Could you check a few things on this model? Use its own coordinates, in mm. Round coordinates to 2 decimals unless told otherwise and drop trailing zeros. Loops run counter-clockwise (first coordinate to the right, second up) from the corner with the lowest first, then second, coordinate; pieces in that order, holes last. Notation, with made-up numbers: M 86.25,58 L 90.25,58 A10 cw 90.25,68 Z; hole C -17.75,-27 d4. An arc over 180 degrees is marked long. Answer in a Markdown table with one row per item.
```python
from build123d import *

# Parameters (mm, degrees)
SKETCH1_R           = 40
SKETCH1_R_2         = 4.1
SKETCH1_R_3         = 1
SKETCH1_R_4         = 2.5
BOSS_EXTRUDE1_DEPTH = 3.175


with BuildPart() as part:
    # Sketch1 → Boss-Extrude1 (new body)
    with BuildSketch(Plane.XY):
        Circle(SKETCH1_R)
        Circle(SKETCH1_R_2, mode=Mode.SUBTRACT)
        with Locations((10, 0)):
            Circle(SKETCH1_R_3, mode=Mode.SUBTRACT)
        with Locations((0, -10)):
            Circle(SKETCH1_R_3, mode=Mode.SUBTRACT)
        with Locations((-10, 0)):
            Circle(SKETCH1_R_3, mode=Mode.SUBTRACT)
        with Locations((0, 10)):
            Circle(SKETCH1_R_3, mode=Mode.SUBTRACT)
        with Locations((0, 32.500000024)):
            Circle(SKETCH1_R_4, mode=Mode.SUBTRACT)
        with Locations((32.500000024, 0)):
            Circle(SKETCH1_R_4, mode=Mode.SUBTRACT)
        with Locations((0, -32.500000024)):
            Circle(SKETCH1_R_4, mode=Mode.SUBTRACT)
        with Locations((-32.500000024, 0)):
            Circle(SKETCH1_R_4, mode=Mode.SUBTRACT)
        with BuildLine():
            ThreePointArc((1.892882879, 15.429065651), (16.987986018, 13.094493375), (30.244053834, 5.505749571))
            ThreePointArc((30.244053834, 5.505749571), (30.545302534, 3.644891179), (28.754168977, 3.057196265))
            ThreePointArc((28.754168977, 3.057196265), (16.369486394, 10.54396404), (2.033129259, 12.519038334))
            ThreePointArc((2.033129259, 12.519038334), (0.481040246, 13.902629865), (1.892882879, 15.429065651))
        make_face(mode=Mode.SUBTRACT)
        with BuildLine():
            ThreePointArc((15.429065651, -1.892882879), (13.094493375, -16.987986018), (5.505749571, -30.244053834))
            ThreePointArc((5.505749571, -30.244053834), (3.644891179, -30.545302534), (3.057196265, -28.754168977))
            ThreePointArc((3.057196265, -28.754168977), (10.54396404, -16.369486394), (12.519038334, -2.033129259))
            ThreePointArc((12.519038334, -2.033129259), (13.902629865, -0.481040246), (15.429065651, -1.892882879))
        make_face(mode=Mode.SUBTRACT)
        with BuildLine():
            ThreePointArc((-1.892882879, -15.429065651), (-16.987986018, -13.094493375), (-30.244053834, -5.505749571))
            ThreePointArc((-30.244053834, -5.505749571), (-30.545302534, -3.644891179), (-28.754168977, -3.057196265))
            ThreePointArc((-28.754168977, -3.057196265), (-16.369486394, -10.54396404), (-2.033129259, -12.519038334))
            ThreePointArc((-2.033129259, -12.519038334), (-0.481040246, -13.902629865), (-1.892882879, -15.429065651))
        make_face(mode=Mode.SUBTRACT)
        with BuildLine():
            ThreePointArc((-15.429065651, 1.892882879), (-13.094493375, 16.987986018), (-5.505749571, 30.244053834))
            ThreePointArc((-5.505749571, 30.244053834), (-3.644891179, 30.545302534), (-3.057196265, 28.754168977))
            ThreePointArc((-3.057196265, 28.754168977), (-10.54396404, 16.369486394), (-12.519038334, 2.033129259))
            ThreePointArc((-12.519038334, 2.033129259), (-13.902629865, 0.481040246), (-15.429065651, 1.892882879))
        make_face(mode=Mode.SUBTRACT)
    extrude(amount=BOSS_EXTRUDE1_DEPTH)


solid = part.part
```
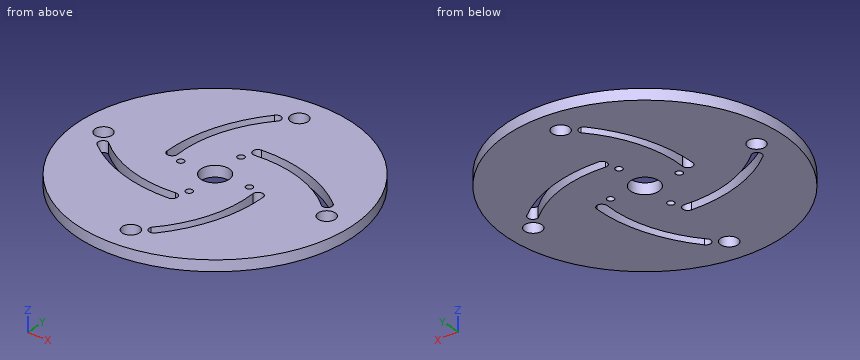
1) I need wall thicknesses on line 1 (Y direction, x = 0, z = 1.45); line 2 (Y direction, x = 10, z = 1.05); line 3 (Y direction, x = -10, z = 2.1). Which ranges of each line are inside material? Lowest first, please.
Computed:
| item | result |
|---|---|
| line 1 | y = -40 to -35, -30 to -11, -9 to -4.1, 4.1 to 9, 11 to 30, 35 to 40 |
| line 2 | y = -38.73 to -23.81, -17.81 to -1, 1 to 12.16, 14.88 to 38.73 |
| line 3 | y = -38.73 to -14.88, -12.16 to -1, 1 to 17.81, 23.81 to 38.73 |
2) I want a section at C-C, the plane z = 2.1. State how many separate pieces and enclosed holes the cut face has, plus the area to 3 significant figures.
Computed:
| item | result |
|---|---|
| separate pieces | 1 |
| enclosed holes | 13 |
| area | 4,540 mm² |
3) I want a section at A-A, the plane y = -10. Please give me the cut outline in (x, z) (3 decimals), plus the area to 3 significant figures.
Computed:
| item | result |
|---|---|
| outline | M -38.73,0 L -23.805,0 L -23.805,3.175 L -38.73,3.175 Z; M -17.807,0 L -1,0 L -1,3.175 L -17.807,3.175 Z; M 1,0 L 12.16,0 L 12.16,3.175 L 1,3.175 Z; M 14.883,0 L 38.73,0 L 38.73,3.175 L 14.883,3.175 Z |
| area | 212 mm² |
4) I want a section at D-D, the plane y = -32.5. Please give me the cut outline in (x, z) (3 decimals).
Computed:
| item | result |
|---|---|
| outline | M -23.318,0 L -2.5,0 L -2.5,3.175 L -23.318,3.175 Z; M 2.5,0 L 23.318,0 L 23.318,3.175 L 2.5,3.175 Z |
5) Will these pins go through, and if not, where does the flat tip stop? P1, Ø6, axis at x = 32.5, y = 0, coming from the +Z side (3 decimals); P2, Ø1, axis at y = 12.5, z = 1, coming from the -X side.
Computed:
| item | result |
|---|---|
| P1 | stops at z = 3.175 |
| P2 | stops at x = -38.16 |
